from build123d import *

# Parameters (mm, degrees)
BOSS_EXTRUDE1_DEPTH = 56.5
BOSS_EXTRUDE2_DEPTH = 10
SKETCH3_R           = 2.5
BOSS_EXTRUDE3_DEPTH = 10


with BuildPart() as part:
    # Sketch1 → Boss-Extrude1 (new body, symmetric)
    with BuildSketch(Plane(origin=(0, 0, 0), x_dir=(0, 0, -1), z_dir=(1, 0, 0))):
        with BuildLine():
            Line((-11, 11.5), (11, 11.5))
            ThreePointArc((11, 11.5), (22.5, 0), (11, -11.5))
            Line((11, -11.5), (-11, -11.5))
            ThreePointArc((-11, -11.5), (-22.5, 0), (-11, 11.5))
        make_face()
    extrude(amount=BOSS_EXTRUDE1_DEPTH, both=True)

    # Sketch2 → Boss-Extrude2 (add)
    with BuildSketch(Plane(origin=(56.5, 0, 0), x_dir=(0, 0, -1), z_dir=(1, 0, 0))):
        with BuildLine():
            Line((-11, 12), (11, 12))
            ThreePointArc((11, 12), (23, 0), (11, -12))
            Line((11, -12), (-11, -12))
            ThreePointArc((-11, -12), (-23, 0), (-11, 12))
        make_face()
    boss_extrude2 = extrude(amount=BOSS_EXTRUDE2_DEPTH)

    # Mirror1: Boss-Extrude2 across plane
    add(boss_extrude2.mirror(Plane(origin=(0, 0, 0), x_dir=(0, 0, 1), z_dir=(1, 0, 0))))

    # Sketch3 → Boss-Extrude3 (add)
    with BuildSketch(Plane(origin=(66.5, 0, 0), x_dir=(0, 0, -1), z_dir=(1, 0, 0))):
        with Locations((-2.7, 0)):
            Circle(SKETCH3_R)
        with Locations((2.7, 0)):
            Circle(SKETCH3_R)
    extrude(amount=BOSS_EXTRUDE3_DEPTH)


solid = part.part
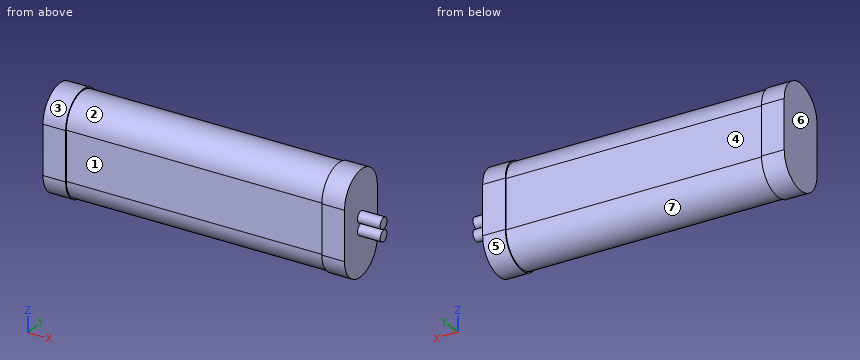
CAD build for the part. Positions are in the model's coordinates, mm. Face numbers are marked on the shaded views. A direction names the side the tool comes from. Round coordinates to 2 decimals unless told otherwise and drop trailing zeros. Write each loop counter-clockwise with the first axis right and the second up, starting at its lowest first coordinate (ties: lowest second). Pieces come first, ordered by that corner, then holes. Notation, with made-up numbers: (76, -7) -> (135, -7) arc R11 ccw to (135, -2) -> close; hole circle Ø3 at (70, -8). An arc over 180 degrees is marked (long way). Answer as a JSON object with one key per item and string values.
(1) Band-saw the part on B-B, the plane z = 2.7. List the corners of the cut face in (x, y), then the cut area to 3 significant figures.
Reported:
{"outline": "(-66.5, -12) -> (-56.5, -12) -> (-56.5, -11.5) -> (56.5, -11.5) -> (56.5, -12) -> (66.5, -12) -> (66.5, -2.5) -> (76.5, -2.5) -> (76.5, 2.5) -> (66.5, 2.5) -> (66.5, 12) -> (56.5, 12) -> (56.5, 11.5) -> (-56.5, 11.5) -> (-56.5, 12) -> (-66.5, 12) -> close", "area": "3,130 mm^2"}
(2) Band-saw the part on A-A, the plane y = 0. List the corners of the cut face in (x, z), then the cut area to 4 significant figures.
Reported:
{"outline": "(-66.5, -23) -> (-56.5, -23) -> (-56.5, -22.5) -> (56.5, -22.5) -> (56.5, -23) -> (66.5, -23) -> (66.5, -5.2) -> (76.5, -5.2) -> (76.5, -0.2) -> (66.5, -0.2) -> (66.5, 0.2) -> (76.5, 0.2) -> (76.5, 5.2) -> (66.5, 5.2) -> (66.5, 23) -> (56.5, 23) -> (56.5, 22.5) -> (-56.5, 22.5) -> (-56.5, 23) -> (-66.5, 23) -> close", "area": "6,105 mm^2"}
(3) Band-saw the part on C-C, the plane x = -58. List the corners of the cut face in (y, z), then the cut area to 3 significant figures.
Reported:
{"outline": "(-12, -11) arc R12 ccw to (12, -11) -> (12, 11) arc R12 ccw to (-12, 11) -> close", "area": "980 mm^2"}
(4) Pin check, flat tips, straight feed: P1, Ø12, axis at y = 3, z = -0.5, coming from the +X side; P2, Ø1.5, axis at x = 46.5, z = -7, coming from the -Y side; P3, Ø2, axis at x = -12.5, z = 2, coming from the +Y side; P4, Ø2, axis at x = 34, z = 13.5, coming from the +Y side. Stop position of each tip, or through.
Reported:
{"P1": "stops at x = 76.5", "P2": "stops at y = -11.5", "P3": "stops at y = 11.5", "P4": "stops at y = 11.4"}
(5) Probe probe 1 along Y at (x, z) = (24.5, 0.5); probe 2 along X at (y, z) = (-0.5, 15.5); probe 3 along Z at (x, y) = (67, -1). List the from-to ranges inside material, lowest first. Write a range as [from, to].
Reported:
{"probe 1": "y = [-11.5, 11.5]", "probe 2": "x = [-66.5, 66.5]", "probe 3": "z = [-4.99, -0.41], [0.41, 4.99]"}
(6) Which spindle directions (+Z, -Z, +X, -X, +Y, -Y) get a long thin tool onto all of the face, cutting with end or side? Do the marked faces 1, 2, 3 and 4. Say none if no direction does.
Reported:
{"face 1": "+Z, -Z, -Y", "face 2": "+Z", "face 3": "+Z, +X, -X", "face 4": "+Z, -Z, +Y"}
(7) Band-saw the part on D-D, the plane z = 14. List the corners of the cut face in (x, y), then the cut area to 3 significant figures.
Reported:
{"outline": "(-66.5, -11.62) -> (-56.5, -11.62) -> (-56.5, -11.1) -> (56.5, -11.1) -> (56.5, -11.62) -> (66.5, -11.62) -> (66.5, 11.62) -> (56.5, 11.62) -> (56.5, 11.1) -> (-56.5, 11.1) -> (-56.5, 11.62) -> (-66.5, 11.62) -> close", "area": "2,970 mm^2"}
(8) Two-plate mould, pull along X, no slides. Class the marked faces 5, 6 and 7: +X half, -X half, draft (parallel to the pull), parting line (faces both ways), or undercut.
Reported:
{"face 5": "draft", "face 6": "-X half", "face 7": "undercut"}
